Read the model definition and answer for the solid it produces. Units are mm, in the model's axes. Coordinates: 2 decimals unless noted, no trailing zeros. Order: outer loops, then holes, each group sorted by start corner. A loop starts at its lowest first (then second) coordinate and runs counter-clockwise, first axis right, second up. Notation, with made-up numbers: (74.25, 0) -> (116.25, 0) arc R18 cw to (116.25, 27) -> close; hole circle Ø2 at (12, 37.25). An arc over 180 degrees is marked (long way). Answer as a JSON object with one key per item and string values. Group by question number.
1) Section A-A on x = 2.5 is taken. Determine the outline of the cut face in (y, z).
2) Consider L1, parallel to X at y = 0.2, z = 10.5; L2, parallel to X at y = 0.4, z = -8.5; L3, parallel to Z at x = -6, y = 0.3. Determine where each line is inside the solid, lowest interval first.
3) Section B-B on z = -26.5 is taken. Determine the outline of the cut face in (x, y), and give its area (3 significant figures).
4) Section D-D on z = -8.5 is taken. Determine the outline of the cut face in (x, y), and give its area (3 significant figures).
5) Given pin 1 (9.5 mm diameter, centred on x = 17.5, z = -8.5, fed in from +Y), flat-ended and moving along its own axis, determine where the tip first touches the part or whether it passes through.
6) Section C-C on y = 0.3 is taken. Count the separate pieces of the cut face and the enclosed holes in it, and give its area (3 significant figures).
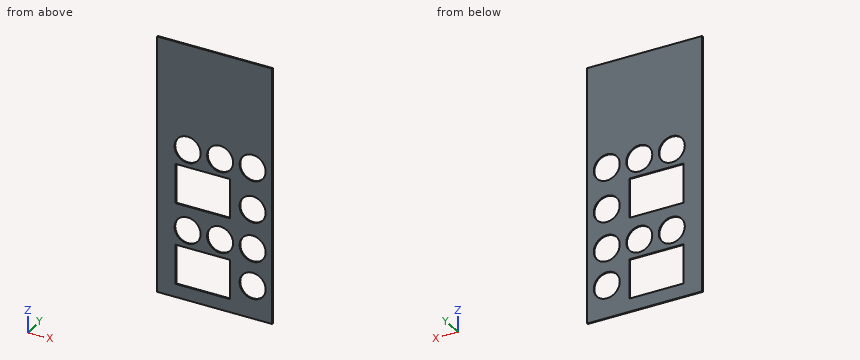
from build123d import *

# Parameters (mm, degrees)
SKETCH_1_W          = 53
SKETCH_1_H          = 117
EXTRUDE_1_DEPTH     = 0.5
SKETCH_2_W          = 25
SKETCH_2_H          = 18
CUT_EXTRUDE_1_DEPTH = 65.224216616
SKETCH_4_R          = 6
CUT_EXTRUDE_2_DEPTH = 65.224216616


with BuildPart() as part:
    # Эскиз1 → Бобышка-Вытянуть1 (new body)
    with BuildSketch(Plane(origin=(0, 0, 0), x_dir=(1, 0, 0), z_dir=(0, 1, 0))):
        Rectangle(SKETCH_1_W, SKETCH_1_H)
    extrude(amount=EXTRUDE_1_DEPTH)

    # Эскиз2 → Вырез-Вытянуть1 (cut, through all)
    with BuildSketch(Plane(origin=(0, 0.5, 0), x_dir=(1, 0, 0), z_dir=(0, 1, 0))):
        with Locations((-5.5, 43.5)):
            Rectangle(SKETCH_2_W, SKETCH_2_H)
        with Locations((-5.5, 6.5)):
            Rectangle(SKETCH_2_W, SKETCH_2_H)
    extrude(amount=-CUT_EXTRUDE_1_DEPTH, mode=Mode.SUBTRACT)

    # Эскиз4 → Вырез-Вытянуть2 (cut, through all)
    with BuildSketch(Plane(origin=(0, 0.5, 0), x_dir=(1, 0, 0), z_dir=(0, 1, 0))):
        with Locations(Location((17.5, 43.5, 0), (0, 0, 270))):
            Circle(SKETCH_4_R)
        with Locations(Location((17.5, 26.5, 0), (0, 0, 270))):
            Circle(SKETCH_4_R)
        with Locations(Location((17.5, 8.5, 0), (0, 0, 270))):
            Circle(SKETCH_4_R)
        with Locations(Location((17.5, -10.5, 0), (0, 0, 270))):
            Circle(SKETCH_4_R)
        with Locations(Location((2.5, 26.5, 0), (0, 0, 270))):
            Circle(SKETCH_4_R)
        with Locations(Location((-12.5, 26.5, 0), (0, 0, 270))):
            Circle(SKETCH_4_R)
        with Locations(Location((2.5, -10.5, 0), (0, 0, 270))):
            Circle(SKETCH_4_R)
        with Locations(Location((-12.5, -10.5, 0), (0, 0, 270))):
            Circle(SKETCH_4_R)
    extrude(amount=-CUT_EXTRUDE_2_DEPTH, mode=Mode.SUBTRACT)


solid = part.part
Worked answers:
{
 "1": {"outline": "(0, -58.5) -> (0.5, -58.5) -> (0.5, -52.5) -> (0, -52.5) -> close; (0, -34.5) -> (0.5, -34.5) -> (0.5, -32.5) -> (0, -32.5) -> close; (0, -20.5) -> (0.5, -20.5) -> (0.5, -15.5) -> (0, -15.5) -> close; (0, 2.5) -> (0.5, 2.5) -> (0.5, 4.5) -> (0, 4.5) -> close; (0, 16.5) -> (0.5, 16.5) -> (0.5, 58.5) -> (0, 58.5) -> close"},
 "2": {"L1": "x = -26.5 to -18.5, -6.5 to -3.5, 8.5 to 11.5, 23.5 to 26.5", "L2": "x = -26.5 to -18, 7 to 11.5, 23.5 to 26.5", "L3": "z = -58.5 to -52.5, -34.5 to -15.5, 2.5 to 58.5"},
 "3": {"outline": "(-26.5, 0) -> (-18.5, 0) -> (-18.5, 0.5) -> (-26.5, 0.5) -> close; (-6.5, 0) -> (-3.5, 0) -> (-3.5, 0.5) -> (-6.5, 0.5) -> close; (8.5, 0) -> (11.5, 0) -> (11.5, 0.5) -> (8.5, 0.5) -> close; (23.5, 0) -> (26.5, 0) -> (26.5, 0.5) -> (23.5, 0.5) -> close", "area": "8.50 mm²"},
 "4": {"outline": "(-26.5, 0) -> (-18, 0) -> (-18, 0.5) -> (-26.5, 0.5) -> close; (7, 0) -> (11.5, 0) -> (11.5, 0.5) -> (7, 0.5) -> close; (23.5, 0) -> (26.5, 0) -> (26.5, 0.5) -> (23.5, 0.5) -> close", "area": "8.00 mm²"},
 "5": {"pin 1": "passes through"},
 "6": {"separate pieces": "1", "enclosed holes": "10", "area": "4,400 mm²"}
}
